```python
from build123d import *

# Parameters (mm, degrees)
PAD_DEPTH    = 8
SKETCH_W     = 4.72
SKETCH_H     = 153.5
PAD001_DEPTH = 5
PAD003_DEPTH = 8


with BuildPart() as part:
    # Sketch003 → Pad (new body)
    with BuildSketch(Plane.XY):
        with BuildLine():
            Line((-1, 0), (-1, 153))
            ThreePointArc((-1, 153), (-1.472972, 154.593853), (-2.36, 156))
            Line((-2.36, 156), (-2.86, 156))
            ThreePointArc((-6, 10), (-3.658792, 82.983414), (-2.86, 156))
            Line((-6, 10), (-6, 2.5))
            Line((-4, 2.5), (-6, 2.5))
            Line((-4, 0), (-4, 2.5))
            Line((-4, 0), (-1, 0))
        make_face()
    extrude(amount=PAD_DEPTH)

    # Sketch → Pad001 (join)
    with BuildSketch(Plane.XY):
        with Locations((0, 79.25)):
            Rectangle(SKETCH_W, SKETCH_H)
    extrude(amount=PAD001_DEPTH)

    # Sketch011 → Pad003 (join)
    with BuildSketch(Plane.XY):
        with BuildLine():
            Line((1, 0), (10, 0))
            Line((10, 0), (10, 10.5))
            ThreePointArc((10, 10.5), (7.593861, 83.266042), (4.36, 156))
            Line((4.36, 156), (2.36, 156))
            ThreePointArc((2.36, 156), (1.472972, 154.593853), (1, 153))
            Line((1, 153), (1, 0))
        make_face()
    extrude(amount=PAD003_DEPTH)


solid = part.part
```
Part model, mm, in its own coordinate system. A direction names the side the tool comes from. Coordinates: 2 decimals unless noted, no trailing zeros. Write each loop counter-clockwise with the first axis right and the second up, starting at its lowest first coordinate (ties: lowest second). Pieces come first, ordered by that corner, then holes.
Item 1: Slice it at D-D (y = 71). Write the cut outline in (x, z).
Item 2: Mould opens along X. For faces 1 (the face through (1, 77, 6)), 2 (the face through (-3.68, 81.96, 3.94)), 3 (the face through (0.7, 79.6, 5)), 4 (the face through (2, 62, 0)) say: released by +X, released by -X, zero draft, split by the parting line, or undercut.
Item 3: Slice it at B-B (y = 133). Write the cut outline in (x, z).
Item 4: Which spindle directions (+Z, -Z, +X, -X, +Y, -Y) get a long thin tool onto all of the face, cutting with end or side? Do faces 5 (the face through (1.483, 154.615, 6.479)), 6 (the face through (-4, 1, 4)), 7 (the face through (-3, 62, 8)). Say none if no direction does.
Item 5: Slice it at A-A (z = 6.25). Write the cut outline in (x, y), and give its area (3 significant figures).
Item 6: Pin check, flat tips, straight feed: pin 1 (1 mm diameter, centred on x = 0, z = 2, fed in from -Y); pin 2 (0.8 mm diameter, centred on y = 1, z = 3, fed in from -X); pin 3 (1.5 mm diameter, centred on y = 122, z = 3.5, fed in from -X). Stop position of each tip, or through.
Item 7: Probe line 1 (Z direction, x = -0.5, y = 89); line 2 (X direction, y = 102, z = 7); line 3 (Y direction, x = 0, z = 4.75). List the from-to ranges inside material, lowest first.
Results found:
1. outline: (-3.94, 0) - (8.06, 0) - (8.06, 8) - (1, 8) - (1, 5) - (-1, 5) - (-1, 8) - (-3.94, 8) - close
2. face 1: undercut
2. face 2: released by -X
2. face 3: undercut
2. face 4: zero draft
3. outline: (-2.95, 0) - (5.47, 0) - (5.47, 8) - (1, 8) - (1, 5) - (-1, 5) - (-1, 8) - (-2.95, 8) - close
4. face 5: +Z, +Y
4. face 6: +Z, -Z, -X, -Y
4. face 7: +Z, +X, -X, +Y, -Y
5. outline: (-6, 2.5) - (-4, 2.5) - (-4, 0) - (-1, 0) - (-1, 153) arc R6.08 ccw to (-2.36, 156) - (-2.86, 156) arc R3456.15 cw to (-6, 10) - close; (1, 0) - (10, 0) - (10, 10.5) arc R6399.14 ccw to (4.36, 156) - (2.36, 156) arc R6.08 ccw to (1, 153) - close
5. area: 1,500 mm2
6. pin 1: stops at y = 2.5
6. pin 2: stops at x = -4
6. pin 3: stops at x = -3.05
7. line 1: z = 0 to 5
7. line 2: x = -3.3 to -1, 1 to 6.84
7. line 3: y = 2.5 to 156
